from build123d import *

# Parameters (mm, degrees)
BOSS_EXTRUDE1_DEPTH = 35
CUT_EXTRUDE1_REACH  = 163.307
SKETCH2_W           = 42
SKETCH2_H           = 21
SKETCH3_R           = 2
CUT_EXTRUDE2_DEPTH  = 10
FILLET1_R           = 20
CUT_EXTRUDE5_REACH  = 163.307
SKETCH6_W           = 42
SKETCH6_H           = 9
SKETCH7_R           = 2
CUT_EXTRUDE6_DEPTH  = 10
CUT_EXTRUDE7_DEPTH  = 9
SKETCH9_R           = 2
CUT_EXTRUDE8_DEPTH  = 10
CUT_EXTRUDE9_DEPTH  = 6
SKETCH11_R          = 2
CUT_EXTRUDE10_DEPTH = 9
SKETCH12_R          = 2
CUT_EXTRUDE11_DEPTH = 10


with BuildPart() as part:
    # Sketch1 → Boss-Extrude1 (new body)
    with BuildSketch(Plane(origin=(0, 0, 0), x_dir=(1, 0, 0), z_dir=(0, 1, 0))):
        Polygon((-38.317617866, 43.23325062), (45.682382134, 43.23325062), (45.682382134, -16.76674938), (65.682382134, -16.76674938), (65.682382134, 118.23325062), (45.682382134, 118.23325062), (45.682382134, 58.23325062), (-38.317617866, 58.23325062), align=None)
    extrude(amount=BOSS_EXTRUDE1_DEPTH)

    # Sketch2 → Cut-Extrude1 (cut, up to next)
    with BuildSketch(Plane(origin=(65.682382134, 0, 0), x_dir=(0, 0, -1), z_dir=(1, 0, 0)), mode=Mode.PRIVATE) as cut_extrude1_sk1:
        with Locations((13.23325062, 19.5)):
            Rectangle(SKETCH2_W, SKETCH2_H)
    cut_extrude1_tool1 = extrude(cut_extrude1_sk1.sketch, amount=-CUT_EXTRUDE1_REACH, mode=Mode.PRIVATE) & part.part
    # Sketch2 → Cut-Extrude1 (cut, up to next)
    with BuildSketch(Plane(origin=(65.682382134, 0, 0), x_dir=(0, 0, -1), z_dir=(1, 0, 0)), mode=Mode.PRIVATE) as cut_extrude1_sk2:
        with Locations((88.23325062, 19.5)):
            Rectangle(SKETCH2_W, SKETCH2_H)
    cut_extrude1_tool2 = extrude(cut_extrude1_sk2.sketch, amount=-CUT_EXTRUDE1_REACH, mode=Mode.PRIVATE) & part.part
    add(cut_extrude1_tool1.solids().sort_by_distance((65.682382, 19.5, -13.233251))[0], mode=Mode.SUBTRACT)
    add(cut_extrude1_tool2.solids().sort_by_distance((65.682382, 19.5, -88.233251))[0], mode=Mode.SUBTRACT)

    # Sketch3 → Cut-Extrude2 (cut)
    with BuildSketch(Plane.ZY.offset(-45.682382134)):
        with Locations((11.26674938, 24.75)):
            Circle(SKETCH3_R)
        with Locations((11.26674938, 15.25)):
            Circle(SKETCH3_R)
        with Locations((-37.73325062, 24.75)):
            Circle(SKETCH3_R)
        with Locations((-37.73325062, 15.25)):
            Circle(SKETCH3_R)
        with Locations(Location((-112.73325062, 24.75, 0), (0, 0, 180))):
            Circle(SKETCH3_R)
        with Locations(Location((-112.73325062, 15.25, 0), (0, 0, 180))):
            Circle(SKETCH3_R)
        with Locations(Location((-63.73325062, 15.25, 0), (0, 0, 180))):
            Circle(SKETCH3_R)
        with Locations(Location((-63.73325062, 24.75, 0), (0, 0, 180))):
            Circle(SKETCH3_R)
    extrude(amount=-CUT_EXTRUDE2_DEPTH, mode=Mode.SUBTRACT)

    # Fillet1
    fillet1_edges = [part.edges().sort_by_distance(p)[0] for p in [
        (55.682382134, 0, -118.23325062),
        (55.682382134, 0, 16.76674938),
    ]]
    fillet(fillet1_edges, radius=FILLET1_R)

    # Sketch6 → Cut-Extrude5 (cut, up to next)
    with BuildSketch(Plane(origin=(65.682382134, 0, 0), x_dir=(0, 0, -1), z_dir=(1, 0, 0)), mode=Mode.PRIVATE) as cut_extrude5_sk1:
        with Locations((13.23325062, 4.5)):
            Rectangle(SKETCH6_W, SKETCH6_H)
    cut_extrude5_tool1 = extrude(cut_extrude5_sk1.sketch, amount=-CUT_EXTRUDE5_REACH, mode=Mode.PRIVATE) & part.part
    # Sketch6 → Cut-Extrude5 (cut, up to next)
    with BuildSketch(Plane(origin=(65.682382134, 0, 0), x_dir=(0, 0, -1), z_dir=(1, 0, 0)), mode=Mode.PRIVATE) as cut_extrude5_sk2:
        with Locations((88.23325062, 4.5)):
            Rectangle(SKETCH6_W, SKETCH6_H)
    cut_extrude5_tool2 = extrude(cut_extrude5_sk2.sketch, amount=-CUT_EXTRUDE5_REACH, mode=Mode.PRIVATE) & part.part
    add(cut_extrude5_tool1.solids().sort_by_distance((65.682382, 4.5, -13.233251))[0], mode=Mode.SUBTRACT)
    add(cut_extrude5_tool2.solids().sort_by_distance((65.682382, 4.5, -88.233251))[0], mode=Mode.SUBTRACT)

    # Sketch7 → Cut-Extrude6 (cut)
    with BuildSketch(Plane.ZY.offset(38.317617866)):
        with Locations((-50.73325062, 25)):
            Circle(SKETCH7_R)
        with Locations((-50.73325062, 10)):
            Circle(SKETCH7_R)
    extrude(amount=-CUT_EXTRUDE6_DEPTH, mode=Mode.SUBTRACT)

    # Sketch8 → Cut-Extrude7 (cut)
    with BuildSketch(Plane.XZ):
        Polygon((45.682382134, -67.23325062), (45.682382134, -58.23325062), (25.682382134, -58.23325062), (25.682382134, -43.23325062), (45.682382134, -43.23325062), (45.682382134, -34.23325062), (65.682382134, -34.23325062), (65.682382134, -67.23325062), align=None)
    extrude(amount=-CUT_EXTRUDE7_DEPTH, mode=Mode.SUBTRACT)

    # Sketch9 → Cut-Extrude8 (cut)
    with BuildSketch(Plane.XZ.offset(-9)):
        with Locations(Location((55.682382134, -42.23325062, 0), (0, 0, 270))):
            Circle(SKETCH9_R)
        with Locations(Location((55.682382134, -59.23325062, 0), (0, 0, 270))):
            Circle(SKETCH9_R)
        with Locations(Location((35.682382134, -50.73325062, 0), (0, 0, 270))):
            Circle(SKETCH9_R)
    extrude(amount=-CUT_EXTRUDE8_DEPTH, mode=Mode.SUBTRACT)

    # Sketch10 → Cut-Extrude9 (cut)
    with BuildSketch(Plane(origin=(0, 35, 0), x_dir=(1, 0, 0), z_dir=(0, 1, 0))):
        Polygon((45.682382134, 62.23325062), (65.682382134, 62.23325062), (65.682382134, 39.23325062), (45.682382134, 39.23325062), (45.682382134, 43.23325062), (31.682382134, 43.23325062), (31.682382134, 58.23325062), (45.682382134, 58.23325062), align=None)
    extrude(amount=-CUT_EXTRUDE9_DEPTH, mode=Mode.SUBTRACT)

    # Sketch11 → Cut-Extrude10 (cut)
    with BuildSketch(Plane(origin=(0, 29, 0), x_dir=(1, 0, 0), z_dir=(0, 1, 0))):
        with Locations(Location((55.682382134, 58.23325062, 0), (0, 0, 270))):
            Circle(SKETCH11_R)
        with Locations(Location((55.682382134, 43.23325062, 0), (0, 0, 270))):
            Circle(SKETCH11_R)
        with Locations(Location((39.682382134, 50.73325062, 0), (0, 0, 270))):
            Circle(SKETCH11_R)
    extrude(amount=-CUT_EXTRUDE10_DEPTH, mode=Mode.SUBTRACT)

    # Sketch12 → Cut-Extrude11 (cut)
    with BuildSketch(Plane(origin=(0, 35, 0), x_dir=(1, 0, 0), z_dir=(0, 1, 0))):
        with Locations(Location((60.682382134, -11.76674938, 0), (0, 0, 270))):
            Circle(SKETCH12_R)
        with Locations(Location((60.682382134, 113.23325062, 0), (0, 0, 270))):
            Circle(SKETCH12_R)
    extrude(amount=-CUT_EXTRUDE11_DEPTH, mode=Mode.SUBTRACT)


solid = part.part
Can you work these out from the model? Positions are in its coordinate system, mm. A direction names the side the tool comes from. Give positions to 0.01 mm unless a question says otherwise; leave off trailing zeros. Write each loop counter-clockwise with the first axis right and the second up, starting at its lowest first coordinate (ties: lowest second). Pieces come first, ordered by that corner, then holes. Notation, with made-up numbers: (-33, 86.25) -> (-7, 86.25) arc R13 cw to (-7, 110.25) -> close; hole circle Ø3 at (67.5, 54.5). An arc over 180 degrees is marked (long way). Answer as a JSON object with one key per item and string values. Group by question number.
Item 1: Suppose I cut it at A-A (y = 32.5). Please give me the cut outline in (x, z), plus the area to 3 significant figures.
Item 2: We'd pull the mould along Y, two halves only. Please class faces 1 (the face through (-33.39, 10.09, -52.73)), 2 (the face through (56, 19, -34.233)), 3 (the face through (50, 9, -51)), 4 (the face through (55.682, 25, -38)): +Y half, -Y half, draft (parallel to the pull), parting line (faces both ways), or undercut.
Item 3: Please list where these lines run through material, in increasing order: line 1 (X direction, y = 26, z = -51); line 2 (Z direction, x = 59, y = 19); line 3 (Z direction, x = 58, y = 32.5). Write a range as [from, to].
Item 4: Suppose I cut it at C-C (x = 11.5). Please give me the cut outline in (y, z).
Item 5: Suppose I cut it at D-D (y = 15.25). State how many separate pieces and enclosed holes the cut face has, plus the area to 3 significant figures.
Item 6: For faces 5 (the face through (50.612, 15.851, 13.174)), 6 (the face through (53.73, 24.56, -58.67)), 7 (the face through (3, 17, -43.233)), which set-ups out of +Z, -Z, +X, -X, +Y, -Y let a thin tool reach every point of the face, with its end or its side?
Item 7: Suppose I cut it at B-B (y = 6). Please give me the cut outline in (x, z), plus the area to 3 significant figures.
Item 8: I'm going to push flat-ended pins straight in: P1, Ø3, axis at x = 36, y = 12.5, coming from the +Z side; P2, Ø3, axis at x = 55, z = -44, coming from the +Y side; P3, Ø1.2, axis at y = 16, z = -63.5, coming from the -X side. Where does each tip first touch, or does it pass through?
Findings:
{
 "1": {"outline": "(-38.32, -58.23) -> (31.68, -58.23) -> (31.68, -43.23) -> (-38.32, -43.23) -> close; (45.68, -118.23) -> (65.68, -118.23) -> (65.68, -62.23) -> (45.68, -62.23) -> close; (45.68, -39.23) -> (65.68, -39.23) -> (65.68, 16.77) -> (45.68, 16.77) -> close; hole circle Ø4 at (60.68, -113.23); hole circle Ø4 at (60.68, 11.77)", "area": "3,260 mm²"},
 "2": {"face 1": "undercut", "face 2": "draft", "face 3": "-Y half", "face 4": "undercut"},
 "3": {"line 1": "x = [-28.32, 37.7], [41.66, 65.68]", "line 2": "z = [-118.21, -109.23], [-67.23, -34.23], [7.77, 16.74]", "line 3": "z = [-118.23, -62.23], [-39.23, 16.77]"},
 "4": {"outline": "(0, -58.23) -> (35, -58.23) -> (35, -43.23) -> (0, -43.23) -> close"},
 "5": {"separate pieces": "3", "enclosed holes": "3", "area": "2,060 mm²"},
 "6": {"face 5": "-X", "face 6": "+Y", "face 7": "+Z, -X, +Y, -Y"},
 "7": {"outline": "(-38.32, -58.23) -> (25.68, -58.23) -> (25.68, -43.23) -> (-38.32, -43.23) -> close; (45.68, -112.52) -> (65.68, -112.52) -> (65.68, -109.23) -> (45.68, -109.23) -> close; (45.68, 7.77) -> (65.68, 7.77) -> (65.68, 11.05) -> (45.68, 11.05) -> close", "area": "1,090 mm²"},
 "8": {"P1": "stops at z = -43.23", "P2": "stops at y = 29", "P3": "stops at x = 55.68"}
}
